Could you check a few things on this model? Use its own coordinates, in mm. A direction names the side the tool comes from. Give positions to 0.01 mm unless a question says otherwise; leave off trailing zeros. Write each loop counter-clockwise with the first axis right and the second up, starting at its lowest first coordinate (ties: lowest second). Pieces come first, ordered by that corner, then holes. Notation, with made-up numbers: (82, 35.5) - (140, 35.5) arc R27 ccw to (140, 71.5) - close; hole circle Ø2 at (84.25, 22.5). An arc over 180 degrees is marked (long way). Answer in a Markdown table with one row per item.
Autodesk Inventor part; units mm, degrees
ref_plane "YZ Plane" through (0, 0, 0) normal (1, 0, 0) x (0, 1, 0)
ref_plane "XZ Plane" through (0, 0, 0) normal (0, 1, 0) x (-1, 0, 0)
ref_plane "XY Plane" through (0, 0, 0) normal (0, 0, 1) x (1, 0, 0)
sketch "スケッチ1" plane through (0, 0, 0) normal (0, 0, 1) x (1, 0, 0)
  line L0 (-24, -34.5) -> (24, -34.5)
  line L1 (24, -34.5) -> (24, 34.5)
  line L2 (24, 34.5) -> (-24, 34.5)
  line L3 (-24, 34.5) -> (-24, -34.5)
  line L4 (-24, -34.5) -> (24, 34.5) construction
  line L5 (24, -34.5) -> (-24, 34.5) construction
  point P0 (0, 0)
  dimension "d0" = 48
  dimension "d1" = 69
extrude "押し出し1" add sketch "スケッチ1" along normal mid plane 18
fillet "フィレット1" radius 3 2 edges at (24, 0, -9) (-24, 0, -9)
fillet "フィレット2" radius 1.5 2 edges at (24, 0, 9) (-24, 0, 9)
fillet "フィレット3" radius 1 16 edges at (-23.5607, 34.5, 8.5607) (-24, 34.5, 0.75) (-23.1213, 34.5, -8.1213) (0, 34.5, -9) (23.1213, 34.5, -8.1213) (24, 34.5, 0.75) (23.5607, 34.5, 8.5607) (0, 34.5, 9) (23.5607, -34.5, 8.5607) (24, -34.5, 0.75) (23.1213, -34.5, -8.1213) (0, -34.5, -9) (-23.1213, -34.5, -8.1213) (-24, -34.5, 0.75) (-23.5607, -34.5, 8.5607) (0, -34.5, 9)
sketch "スケッチ2" plane through (0, 0, 9) normal (0, 0, 1) x (1, 0, 0)
  line L0 (8.4, 26.4) -> (17, 26.4)
  line L1 (17, 26.4) -> (17, 31)
  line L2 (17, 31) -> (8.4, 31)
  line L3 (8.4, 31) -> (8.4, 26.4)
  line L4 (8.4, 26.4) -> (17, 31) construction
  line L5 (17, 26.4) -> (8.4, 31) construction
  line L6 (24, -33.5) -> (24, 33.5) construction
  line L7 (22.5, 34.5) -> (-22.5, 34.5) construction
  point P0 (0, 0)
  point P1 (12.7, 28.7)
  dimension "d7" = 7
  dimension "d8" = 3.5
  dimension "d9" = 4.6
  dimension "d10" = 8.6
extrude "押し出し2" cut sketch "スケッチ2" against normal blind 4
sketch "スケッチ3" plane through (0, 0, 5) normal (0, 0, 1) x (1, 0, 0)
  line L0 (17, 31) -> (17, 26.4) construction
  line L1 (8.4, 31) -> (17, 31) construction
  line L2 (8.4, 26.4) -> (8.4, 31) construction
  line L3 (17, 26.4) -> (8.4, 26.4) construction
  line L4 (8.4, 28.7) -> (17, 28.7) construction
  line L5 (12.2, 27.2) -> (9.2, 27.2)
  line L6 (9.2, 27.2) -> (9.2, 30.2)
  line L7 (9.2, 30.2) -> (12.2, 30.2)
  line L8 (12.2, 30.2) -> (12.2, 27.2)
  line L9 (12.2, 27.2) -> (9.2, 30.2) construction
  line L10 (9.2, 27.2) -> (12.2, 30.2) construction
  point P0 (0, 0)
  point P1 (10.7, 28.7)
  dimension "d13" = 3
  dimension "d14" = 3
  dimension "d15" = 0.8
extrude "押し出し3" add sketch "スケッチ3" along normal blind 5.5
properties part number "batt_box"
1) On a 3-axis mill with a long thin cutter (end or side, diameter ignored), from which of +Z, -Z, +X, -X, +Y, -Y can I reach the whole of each face in a straight line? I mean faces 1 (the face through (-23.55, -0.47, 8.57)), 2 (the face through (13, 26.4, 7)). Say none if no direction works.
Check values:
| item | result |
|---|---|
| face 1 | +Z, -X, +Y, -Y |
| face 2 | +Z |
2) If I drill on line 1 (Z direction, x = -2.5, y = 4.5); line 2 (X direction, y = 30, z = 8.25); line 3 (X direction, y = -9.5, z = 8.75), over which ranges is the centre line in solid material (lowest first)?
Check values:
| item | result |
|---|---|
| line 1 | z = -9 to 9 |
| line 2 | x = -23.8 to 8.4, 9.2 to 12.2, 17 to 23.8 |
| line 3 | x = -23.33 to 23.33 |
3) Imagine slicing it at A-A (y = -17). List the corners of the cut face in (x, z) for me, then the cut area to 3 significant figures.
Check values:
| item | result |
|---|---|
| outline | (-24, -6) arc R3 ccw to (-21, -9) - (21, -9) arc R3 ccw to (24, -6) - (24, 7.5) arc R1.5 ccw to (22.5, 9) - (-22.5, 9) arc R1.5 ccw to (-24, 7.5) - close |
| area | 859 mm2 |
4) Will this pin go through, and if not, where does the flat tip stop? P1, Ø1.5, axis at y = 29.5, z = 8.5, coming from the +X side.
Check values:
| item | result |
|---|---|
| P1 | stops at x = 23.98 |
5) Imagine slicing it at B-B (x = -15.5). List the corners of the cut face in (y, z) for me, then the cut area to 3 significant figures.
Check values:
| item | result |
|---|---|
| outline | (-34.5, -8) arc R1 ccw to (-33.5, -9) - (33.5, -9) arc R1 ccw to (34.5, -8) - (34.5, 8) arc R1 ccw to (33.5, 9) - (-33.5, 9) arc R1 ccw to (-34.5, 8) - close |
| area | 1,240 mm2 |
